Work out the finished part from the listing and answer in its coordinate system (mm). A direction names the side the tool comes from. Round coordinates to 2 decimals unless told otherwise and drop trailing zeros. Write each loop counter-clockwise with the first axis right and the second up, starting at its lowest first coordinate (ties: lowest second). Pieces come first, ordered by that corner, then holes. Notation, with made-up numbers: M -24.75,38.5 L 17.25,38.5 A26 ccw 17.25,55.5 Z; hole C 78.25,23 d3. An arc over 180 degrees is marked long. One line per item, written item: value. Start each with the question number.
Q1. The mould has two halves that part along X. Classify faces 1 (the flat face through (-8, -21, 2)), 2 (the cylindrical face through (15.14, 33.1, 2.03)), 3 (the flat face through (-16, 0, 2)): released by +X, released by -X, zero draft, split by the parting line, or undercut.
Q2. Find section C-C (y = 3). Write down the section's boundary in (x, z), and give its area (3 significant figures).
Q3. A tool of negligible diameter and unlimited length cuts with its end or side. For faces 4 (the flat face through (8, -22, 1)), 5 (the cylindrical face through (-6, 28.9, 0.6)), 6 (the cylindrical face through (0.04, 25.14, 3.1)), from which of +Z, -Z, +X, -X, +Y, -Y can it reach the whole face along a straight path? Write none if from no direction.
Q4. Find section A-A (y = 29). Write down the section's boundary in (x, z), and give its area (3 significant figures).
Q5. Consider probe 1 along Y at (x, z) = (0.5, 1); probe 2 along X at (y, z) = (0, 2.65); probe 3 along Y at (x, z) = (-7, 1.2). Determine where each line is inside the solid, lowest interval first.
Q6. Find section B-B (x = 10.5). Write down the section's boundary in (y, z), and give its area (3 significant figures).
Q7. Given pin 1 Ø0.6 at (x, y) = (9.5, 20.5) entering from -Z, flat-ended and moving along its own axis, determine where the tip first touches the part or whether it passes through.
Solid Edge part; units mm, degrees
sketch "Sketch1" plane through (0, 0, 0) normal (0, 0, 1) x (1, 0, 0)
  line L0 (-3, -26) -> (3, -26)
  line L1 (3, -32) -> (-3, -32)
  arc A0 (-3, -32) -> (-3, -26) centre (-3, -29) cw
  arc A1 (3, -26) -> (3, -32) centre (3, -29) cw
  line L2 (-16, -34) -> (-16, 34)
  line L3 (-16, 34) -> (16, 34)
  line L4 (16, 34) -> (16, -34)
  line L5 (16, -34) -> (-16, -34)
  line L6 (12, -20) -> (-12, -20)
  line L7 (-12, -20) -> (-12, 20)
  line L8 (-12, 20) -> (12, 20)
  line L9 (12, 20) -> (12, -20)
  line L10 (3, 32) -> (-3, 32)
  arc A2 (-3, 32) -> (-3, 26) centre (-3, 29) ccw
  line L11 (-3, 26) -> (3, 26)
  arc A3 (3, 26) -> (3, 32) centre (3, 29) ccw
extrude "Protrusion1" add sketch "Sketch1" along normal blind 4
sketch "Sketch2" plane through (0, 0, 0) normal (0, 0, 1) x (1, 0, 0)
  line L0 (4.5, -24) -> (-4.5, -24)
  line L1 (-4.5, -24) -> (-4.5, -20)
  line L2 (-4.5, -20) -> (4.5, -20)
  line L3 (4.5, -20) -> (4.5, -24)
  line L4 (-4.5, 20) -> (4.5, 20)
  line L5 (4.5, 20) -> (4.5, 24)
  line L6 (4.5, 24) -> (-4.5, 24)
  line L7 (-4.5, 24) -> (-4.5, 20)
extrude "ExtrudedCutout_1" cut sketch "Sketch2" along normal blind 3
fillet "Round_1" radius 3 12 edges at (-16, -34, 2) (16, -34, 2) (16, 34, 2) (-16, 34, 2) (0, 26, 4) (6, 29, 4) (0, 32, 4) (-6, 29, 4) (0, -32, 4) (-6, -29, 4) (0, -26, 4) (6, -29, 4)
sketch "Sketch3" plane through (0, 0, 0) normal (0, 0, -1) x (-1, 0, 0)
  line L0 (-12, 22) -> (-4.5, 22)
  line L1 (-4.5, 22) -> (-4.5, 20)
  line L2 (-4.5, 20) -> (-12, 20)
  line L3 (-12, 20) -> (-12, 22)
  line L4 (4.5, 22) -> (12, 22)
  line L5 (12, 22) -> (12, 20)
  line L6 (12, 20) -> (4.5, 20)
  line L7 (4.5, 20) -> (4.5, 22)
  line L8 (-12, -20) -> (-4.5, -20)
  line L9 (-4.5, -20) -> (-4.5, -22)
  line L10 (-4.5, -22) -> (-12, -22)
  line L11 (-12, -22) -> (-12, -20)
  line L12 (12, -20) -> (4.5, -20)
  line L13 (4.5, -20) -> (4.5, -22)
  line L14 (4.5, -22) -> (12, -22)
  line L15 (12, -22) -> (12, -20)
extrude "ExtrudedCutout_2" cut sketch "Sketch3" against normal blind 2
The answers:
1. face 1: undercut
1. face 2: released by +X
1. face 3: released by -X
2. outline: M -16,0 L -12,0 L -12,4 L -16,4 Z; M 12,0 L 16,0 L 16,4 L 12,4 Z
2. area: 32.0 mm2
3. face 4: -Z
3. face 5: +Z, -Z
3. face 6: +Z
4. outline: M -16,0 L -6,0 L -6,1 A3 ccw -9,4 L -16,4 Z; M 6,0 L 16,0 L 16,4 L 9,4 A3 ccw 6,1 Z
4. area: 76.1 mm2
5. probe 1: -34 to -32, -26 to -24, 24 to 26, 32 to 34
5. probe 2: -16 to -12, 12 to 16
5. probe 3: -34 to -22, 22 to 34
6. outline: M -34,0 L -22,0 L -22,2 L -20,2 L -20,4 L -34,4 Z; M 20,2 L 22,2 L 22,0 L 34,0 L 34,4 L 20,4 Z
6. area: 104 mm2
7. pin 1: z = 2
